Read the model definition and answer for the solid it produces. Units are mm, in the model's axes. Coordinates: 2 decimals unless noted, no trailing zeros. Loops run counter-clockwise (first coordinate to the right, second up) from the corner with the lowest first, then second, coordinate; pieces in that order, holes last. Notation, with made-up numbers: (53.25, 13) -> (94.25, 13) arc R21 ccw to (94.25, 34) -> close; hole circle Ø9 at (-27.5, -2.75). An arc over 180 degrees is marked (long way). Answer as a JSON object with one key per item and string values. Group by question number.
1) Consider probe 1 along Y at (x, z) = (0, 5.25); probe 2 along Y at (x, z) = (-1.75, 6.5); probe 3 along X at (y, z) = (-3.5, 7). Determine where each line is inside the solid, lowest interval first. Write a range as [from, to].
2) Section D-D, the plane y = -21 is taken. Give the vertices of the cut face in (x, z).
3) Section A-A, the plane x = 0 is taken. Give the vertices of the cut face in (y, z), plus the area to 3 significant figures.
4) Section C-C, the plane z = 2.75 is taken. Give the vertices of the cut face in (x, y).
5) Flat-ended cylindrical pins translate along their axes: P1, Ø1, axis at y = -5.5, z = 5.5, coming from the -X side; P2, Ø4, axis at x = -3.5, y = -19, coming from the +Z side; P3, Ø1, axis at x = 4, z = 2.5, coming from the +Y side. Find the tip coordinate at first contact, or state that the pin passes through.
from build123d import *

# Parameters (mm, degrees)
SKETCH1_R           = 5.7
SKETCH1_R_2         = 4.2
BOSS_EXTRUDE1_DEPTH = 9.1
SKETCH2_R           = 0.65
BOSS_EXTRUDE2_DEPTH = 48


with BuildPart() as part:
    # Sketch1 → Boss-Extrude1 (new body)
    with BuildSketch(Plane.XY):
        Circle(SKETCH1_R)
        Circle(SKETCH1_R_2, mode=Mode.SUBTRACT)
    extrude(amount=BOSS_EXTRUDE1_DEPTH)

    # Sketch2 → Boss-Extrude2 (add, symmetric)
    with BuildSketch(Plane(origin=(0, 0, 0), x_dir=(1, 0, 0), z_dir=(0, 1, 0))):
        with Locations(Location((-4.94879538, -8.44469772, 0), (0, 0, 90))):
            Circle(SKETCH2_R)
    extrude(amount=BOSS_EXTRUDE2_DEPTH, both=True)


solid = part.part
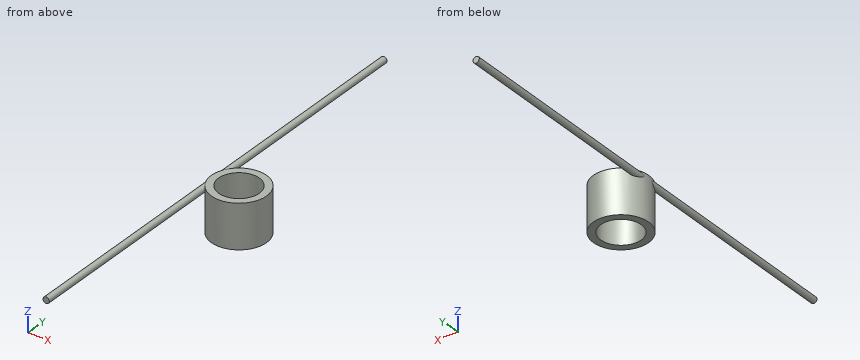
Determined:
{
 "1": {"probe 1": "[-5.7, -4.2], [4.2, 5.7]", "probe 2": "[-5.42, -3.82], [3.82, 5.42]", "probe 3": "[-4.5, -2.32], [2.32, 4.5]"},
 "2": {"outline": "circle Ø1.3 at (-4.95, 8.44)"},
 "3": {"outline": "(-5.7, 0) -> (-4.2, 0) -> (-4.2, 9.1) -> (-5.7, 9.1) -> close; (4.2, 0) -> (5.7, 0) -> (5.7, 9.1) -> (4.2, 9.1) -> close", "area": "27.3 mm²"},
 "4": {"outline": "circle Ø11.4 at (0, 0); hole circle Ø8.4 at (0, 0)"},
 "5": {"P1": "x = -2.74", "P2": "z = 9.09", "P3": "y = 4.5"}
}
